Geometry check sheet. Reference: the model listing, model coordinates, mm. A direction names the side the tool comes from. Round coordinates to 2 decimals unless told otherwise and drop trailing zeros. Order: outer loops, then holes, each group sorted by start corner. A loop starts at its lowest first (then second) coordinate and runs counter-clockwise, first axis right, second up.
(1) Sectioned sample at D-D (y = -5.5). Record the boundary of the cut face in (x, z).
(2) Sectioned sample at A-A (x = 0). Record the boundary of the cut face in (y, z) (3 decimals).
(3) Material ranges on line 1 along Z through (x, y) = (0, 0); line 2 along Z through (x, y) = (0, 6); line 3 along X through (y, z) = (11, -24), recorded low to high.
(4) Set-up check for faces 5 (the face through (15.2, -1, 19)), 6 (the face through (-18, 12.7, -22)), 7 (the face through (2.3, 4.61, -16.8)), 8 (the face through (15.2, 10, -9)): record each of +Z, -Z, +X, -X, +Y, -Y from which the full face is reachable in a straight line by a thin tool's end or side.
(5) Sectioned sample at B-B (y = 8). Record the boundary of the cut face in (x, z).
(6) Go/stop test with flat-tipped pins: pin 1 (3 mm diameter, centred on x = -2, z = 11.5, fed in from +Y); pin 2 (1.9 mm diameter, centred on y = 10.16, z = 14.92, fed in from -X); pin 3 (1.6 mm diameter, centred on x = 16.5, z = -19, fed in from +Y); pin 4 (11.5 mm diameter, centred on x = -2, z = -16.5, fed in from +Y). Record where each tip stops, or that it passes through.
(7) Release check for a two-part mould opening along Y. For faces 1 (the face through (-18.89, 15.54, -5.1)), 2 (the face through (18, 12.7, -22)), 3 (the face through (-17.7, 11.2, -2.7)), 4 (the face through (5.008, 6.004, -20.627)) record: +Y half, -Y half, draft (parallel to the pull), parting line (faces both ways), or undercut.
(8) Sectioned sample at C-C (x = -16). Record the boundary of the cut face in (y, z) (3 decimals), plus the area to 3 significant figures.
from build123d import *

# Parameters (mm, degrees)
SKETCH1_W                       = 45.72
SKETCH1_H                       = 60.96
BOSS_EXTRUDE1_DEPTH             = 6.35
SKETCH2_W                       = 7.6600046
SKETCH2_H                       = 60.96
BOSS_EXTRUDE2_DEPTH             = 20.955
LPATTERN1_COUNT                 = 3
LPATTERN1_PITCH                 = 17.018
SKETCH1_3_W                     = 45.72
SKETCH1_3_H                     = 60.96
BOSS_EXTRUDE3_DEPTH             = 2.54
CUT_EXTRUDE1_START              = 15.199995
SKETCH11_W                      = 60.96
SKETCH11_H                      = 14.3449802
CUT_EXTRUDE1_DEPTH              = 17.78
CUT_EXTRUDE2_DEPTH              = 62.358877312
SKETCH17_W                      = 45.72
SKETCH17_H                      = 60.96
BOSS_EXTRUDE4_DEPTH             = 6.785
SKETCH19_W                      = 30.3999908
SKETCH19_H                      = 60.96
BOSS_EXTRUDE5_DEPTH             = 1.0100056
CBORE_FOR_M5_SBHCS2_D           = 5.5
CBORE_FOR_M5_SBHCS2_CBORE_D     = 10.5
CBORE_FOR_M5_SBHCS2_CBORE_DEPTH = 2.75
CUT_EXTRUDE3_DEPTH              = 82.222264916
CUT_EXTRUDE3_DEPTH_BACK         = 82.222264916
SKETCH24_W                      = 5.08
SKETCH24_H                      = 45.72
SKETCH25_W                      = 7.6600046
SKETCH25_H                      = 36.63
CUT_EXTRUDE4_DEPTH              = 12.7
SKETCH26_W                      = 2.400000026
SKETCH26_H                      = 36.63
CUT_EXTRUDE5_DEPTH              = 67.262485805
SKETCH27_W                      = 2.5
SKETCH27_H                      = 36.63
CUT_EXTRUDE6_DEPTH              = 67.262485805
CHAMFER1_SIZE                   = 2.5


with BuildPart() as part:
    # Sketch1 → Boss-Extrude1 (new body)
    with BuildSketch(Plane(origin=(0, 0, 0), x_dir=(1, 0, 0), z_dir=(0, 1, 0))):
        Rectangle(SKETCH1_W, SKETCH1_H)
    extrude(amount=BOSS_EXTRUDE1_DEPTH)

    # Sketch2 → Boss-Extrude2 (add)
    with BuildSketch(Plane(origin=(0, 6.35, 0), x_dir=(1, 0, 0), z_dir=(0, 1, 0))):
        with Locations((-19.0299977, 0)):
            Rectangle(SKETCH2_W, SKETCH2_H)
        with Locations((19.0299977, 0)):
            Rectangle(SKETCH2_W, SKETCH2_H)
    extrude(amount=BOSS_EXTRUDE2_DEPTH)

    # Sketch7 → M2 Clearance Hole2 (revolve, cut)
    with BuildSketch(Plane(origin=(22.86, 10.16, 14.9171914), x_dir=(0, 0, -1), z_dir=(0, 1, 0))):
        Polygon((0, 0), (0, 46.441032743), (1.2, 45.72), (1.2, 0), align=None)
    m2_clearance_hole2 = revolve(axis=Axis((29.21, 10.16, 14.9171914), (-1, 0, 0)), mode=Mode.SUBTRACT)

    # LPattern1: M2 Clearance Hole2 ×3
    with Locations(*[(0, 0, -i * LPATTERN1_PITCH) for i in range(1, LPATTERN1_COUNT)]):
        add(m2_clearance_hole2, mode=Mode.SUBTRACT)

    # Sketch1<3> → Boss-Extrude3 (add)
    with BuildSketch(Plane(origin=(0, 0, 0), x_dir=(1, 0, 0), z_dir=(0, 1, 0))):
        Rectangle(SKETCH1_3_W, SKETCH1_3_H)
    extrude(amount=-BOSS_EXTRUDE3_DEPTH)

    # Sketch11 → Cut-Extrude1 (cut, symmetric)
    with BuildSketch(Plane.ZY.offset(-15.1999954).offset(CUT_EXTRUDE1_START)):
        with Locations((0, 20.1325099)):
            Rectangle(SKETCH11_W, SKETCH11_H)
    extrude(amount=CUT_EXTRUDE1_DEPTH, both=True, mode=Mode.SUBTRACT)

    # Sketch12 → Cut-Extrude2 (cut, through all)
    with BuildSketch(Plane(origin=(22.86, 0, 0), x_dir=(0, 0, -1), z_dir=(1, 0, 0))):
        with BuildLine():
            Line((13.105000048, 12.7), (30.48, 12.7))
            Line((30.48, 12.7), (30.48, 27.305))
            Line((30.48, 27.305), (25.661312206, 27.305))
            ThreePointArc((25.661312206, 27.305), (3.474748234, 33.679387055), (13.105000048, 12.7))
        make_face()
    extrude(amount=-CUT_EXTRUDE2_DEPTH, mode=Mode.SUBTRACT)

    # Sketch17 → Boss-Extrude4 (add)
    with BuildSketch(Plane.XZ.offset(2.54)):
        Rectangle(SKETCH17_W, SKETCH17_H)
    extrude(amount=BOSS_EXTRUDE4_DEPTH)

    # Sketch19 → Boss-Extrude5 (add)
    with BuildSketch(Plane(origin=(0, 6.35, 0), x_dir=(1, 0, 0), z_dir=(0, 1, 0))):
        Rectangle(SKETCH19_W, SKETCH19_H)
    extrude(amount=BOSS_EXTRUDE5_DEPTH)

    # CBORE for M5 SBHCS2 (through all)
    with Locations(Plane(origin=(0, 7.3600056, 0), x_dir=(1, 0, 0), z_dir=(0, 1, 0))):
        with Locations((0, -12.7), (0, 19.05)):
            CounterBoreHole(CBORE_FOR_M5_SBHCS2_D / 2, CBORE_FOR_M5_SBHCS2_CBORE_D / 2, CBORE_FOR_M5_SBHCS2_CBORE_DEPTH)

    # Sketch24 → Cut-Extrude3 (cut, two sides: drawn at the far end of the back side and taken through both)
    with BuildSketch(Plane(origin=(31.571183672, -12.7, -14.6188086), x_dir=(0, 0, -1), z_dir=(0, 1, 0)).offset(-CUT_EXTRUDE3_DEPTH_BACK)):
        with Locations((-42.5588086, 31.571183672)):
            Rectangle(SKETCH24_W, SKETCH24_H)
    extrude(amount=CUT_EXTRUDE3_DEPTH + CUT_EXTRUDE3_DEPTH_BACK, mode=Mode.SUBTRACT)

    # Sketch25 → Cut-Extrude4 (cut)
    with BuildSketch(Plane.XY.offset(25.4)):
        with Locations((19.0299977, 8.99)):
            Rectangle(SKETCH25_W, SKETCH25_H)
    extrude(amount=-CUT_EXTRUDE4_DEPTH, mode=Mode.SUBTRACT)

    # Sketch26 → Cut-Extrude5 (cut, through all)
    with BuildSketch(Plane.XY.offset(25.4)):
        with Locations((21.659999987, 8.99)):
            Rectangle(SKETCH26_W, SKETCH26_H)
    extrude(amount=-CUT_EXTRUDE5_DEPTH, mode=Mode.SUBTRACT)

    # Sketch27 → Cut-Extrude6 (cut, through all)
    with BuildSketch(Plane.XY.offset(25.4)):
        with Locations((-21.61, 8.99)):
            Rectangle(SKETCH27_W, SKETCH27_H)
    extrude(amount=-CUT_EXTRUDE6_DEPTH, mode=Mode.SUBTRACT)

    # Chamfer1
    chamfer1_edges = [part.edges().sort_by_distance(p)[0] for p in [
        (-20.36, 1.6875, -30.48),
        (-20.36, 8.99, 25.4),
    ]]
    chamfer(chamfer1_edges, length=CHAMFER1_SIZE)


solid = part.part
Answer below:
1. outline: (-20.36, -27.98) - (-17.86, -30.48) - (20.46, -30.48) - (20.46, 12.7) - (15.2, 12.7) - (15.2, 25.4) - (-17.86, 25.4) - (-20.36, 22.9) - close; hole circle Ø5.5 at (0, -19.05); hole circle Ø5.5 at (0, 12.7)
2. outline: (-9.325, -30.48) - (7.36, -30.48) - (7.36, -24.3) - (4.61, -24.3) - (4.61, -21.8) - (-9.325, -21.8) - close; (-9.325, -16.3) - (4.61, -16.3) - (4.61, -13.8) - (7.36, -13.8) - (7.36, 7.45) - (4.61, 7.45) - (4.61, 9.95) - (-9.325, 9.95) - close; (-9.325, 15.45) - (4.61, 15.45) - (4.61, 17.95) - (7.36, 17.95) - (7.36, 25.4) - (-9.325, 25.4) - close
3. line 1: z = -30.48 to -21.8, -16.3 to 9.95, 15.45 to 25.4
3. line 2: z = -30.48 to -24.3, -13.8 to 7.45, 17.95 to 25.4
3. line 3: x = -20.36 to -15.2, 15.2 to 20.46
4. face 5: +Z, +X, +Y, -Y
4. face 6: -Z, +X, -X, +Y
4. face 7: +Y
4. face 8: +Z, -Z, +Y
5. outline: (-20.36, -27.98) - (-17.86, -30.48) - (-15.2, -30.48) - (-15.2, 25.4) - (-17.86, 25.4) - (-20.36, 22.9) - close; (15.2, -30.48) - (20.46, -30.48) - (20.46, 12.7) - (15.2, 12.7) - close
6. pin 1: stops at y = 4.61
6. pin 2: passes through
6. pin 3: stops at y = 12.7
6. pin 4: stops at y = 7.36
7. face 1: undercut
7. face 2: +Y half
7. face 3: undercut
7. face 4: draft
8. outline: (-9.325, -30.48) - (12.7, -30.48) - (12.7, -13.105) arc R12.7 cw to (12.96, -10.548) - (12.96, 25.4) - (-9.325, 25.4) - close; hole circle Ø2.4 at (10.16, -19.119); hole circle Ø2.4 at (10.16, -2.101); hole circle Ø2.4 at (10.16, 14.917)
8. area: 1,230 mm2
